Input: part model. Units: mm. Frame: model coordinates. Face numbers are marked on the shaded views. A direction names the side the tool comes from. Coordinates: 2 decimals unless noted, no trailing zeros. Write each loop counter-clockwise with the first axis right and the second up, starting at its lowest first coordinate (ties: lowest second). Pieces come first, ordered by that corner, then holes. Notation, with made-up numbers: (44.25, 88) - (93.25, 88) arc R21 cw to (93.25, 119) - close; hole circle Ø6 at (54.5, 23.25). An arc over 180 degrees is marked (long way). Put each result on its own line as item: value. Start each with the question number.
1. Cut plane C-C, the plane z = 17. Return loops of the section in (x, y), and give its area (3 significant figures).
2. Cut plane A-A, the plane y = 0. Return loops of the section in (x, z), and give its area (3 significant figures).
3. Line query: line 1 (Y direction, x = 0.75, z = 31); line 2 (X direction, y = -0.15, z = 16.5); line 3 (X direction, y = 2.65, z = 23.5). Output: solid intervals per line, ascending.
4. Access query for the marked faces 1, 2 and 3. Directions: +Z, -Z, +X, -X, +Y, -Y. A direction counts if a zero-diameter tool reaches every point of the face in a straight line with its end or side. Return the directions, or none.
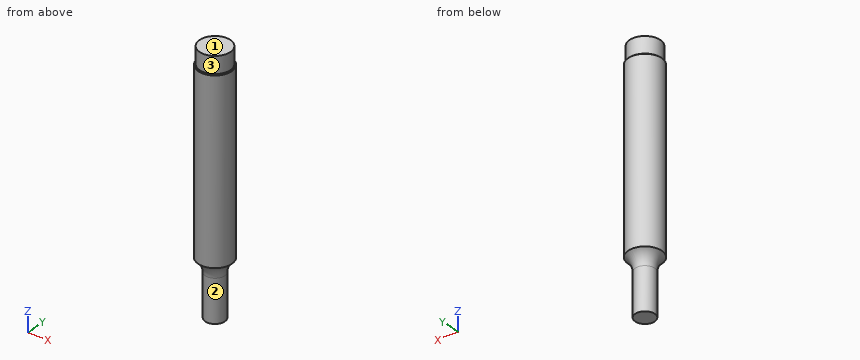
Autodesk Inventor part; units mm, degrees
ref_plane "YZ Plane" through (0, 0, 0) normal (1, 0, 0) x (0, 1, 0)
ref_plane "XZ Plane" through (0, 0, 0) normal (0, 1, 0) x (-1, 0, 0)
ref_plane "XY Plane" through (0, 0, 0) normal (0, 0, 1) x (1, 0, 0)
sketch "Sketch1" plane through (0, 0, 0) normal (0, 0, 1) x (1, 0, 0)
  circle A0 centre (0, 0) radius 3
  dimension "d0" = 6
extrude "Extrusion1" add sketch "Sketch1" along normal blind 32
sketch "Sketch2" plane through (0, 0, 32) normal (0, 0, 1) x (1, 0, 0)
  circle A0 centre (0, 0) radius 2.75
  dimension "d3" = 5.5
extrude "Extrusion2" add sketch "Sketch2" along normal blind 3
sketch "Sketch3" plane through (0, 0, 0) normal (0, 0, -1) x (-1, 0, 0)
  circle A0 centre (0, 0) radius 1.75
  dimension "d6" = 3.5
extrude "Extrusion3" add sketch "Sketch3" along normal blind 10
fillet "Fillet1" radius 3 1 edges at (1.75, 0, 0)
thread "Thread1"
chamfer "Chamfer1" distance 0.1 angle 45 1 edges at (-3, 0, 32)
properties part number "6mm Inductive Probe" material "Stainless Steel"
Report:
1. outline: circle Ø6 at (0, 0)
1. area: 28.3 mm^2
2. outline: (-3, 0) arc R3 cw to (-1.75, -2.44) - (-1.75, -10) - (1.75, -10) - (1.75, -2.44) arc R3 cw to (3, 0) - (3, 31.9) - (2.9, 32) - (2.75, 32) - (2.75, 35) - (-2.75, 35) - (-2.75, 32) - (-2.9, 32) - (-3, 31.9) - close
2. area: 245 mm^2
3. line 1: y = -2.9 to 2.9
3. line 2: x = -3 to 3
3. line 3: x = -1.41 to 1.41
4. face 1: +Z, +X, -X, +Y, -Y
4. face 2: -Z
4. face 3: +Z
